Part model, mm, in its own coordinate system. A direction names the side the tool comes from. Give positions to 0.01 mm unless a question says otherwise; leave off trailing zeros. Order: outer loops, then holes, each group sorted by start corner. A loop starts at its lowest first (then second) coordinate and runs counter-clockwise, first axis right, second up. Notation, with made-up numbers: (75, 60.25) - (116, 60.25) arc R24 ccw to (116, 94.25) - close; hole circle Ø7 at (-2.5, 62). An arc over 180 degrees is marked (long way). One line per item, written item: value.
```python
from build123d import *

# Parameters (mm, degrees)
F1_DEPTH = 63.5
F2_DEPTH = 25.4
F3_DEPTH = 7.9375
F5_R     = 6.35


with BuildPart() as f1:
    # F0 (on Front) → F1 (new body, symmetric)
    with BuildSketch(Plane.XZ):
        Polygon((-41.275, 9.525), (-41.275, -9.525), (41.275, -9.525), (41.275, 9.525), (22.225, 9.525), align=None)
    extrude(amount=F1_DEPTH, both=True)

    # F0 (on Front) → F2 (join, symmetric)
    with BuildSketch(Plane.XZ):
        with BuildLine():
            Line((22.225, 9.525), (41.275, 9.525))
            Line((41.275, 9.525), (41.275, 30.6455698351))
            ThreePointArc((41.275, 30.6455698351), (44.8569757439, 39.2932242561), (53.5046301649, 42.8752))
            Line((53.5046301649, 42.8752), (60.325, 42.8752))
            Line((60.325, 42.8752), (60.325, 61.9252))
            Line((60.325, 61.9252), (53.5046301649, 61.9252))
            add(Edge.make_bspline(
                [(51.2267353125, 61.8421475047), (51.9857307237, 61.8741703131), (52.7450911942, 61.9018592787), (53.5046301649, 61.9252)],
                knots=[106.5779912672, 106.5779912672, 106.5779912672, 106.5779912672, 108.3003197328, 108.3003197328, 108.3003197328, 108.3003197328], degree=3))
            ThreePointArc((51.2267353125, 61.8421475047), (30.595385614, 51.943029246), (22.225, 30.6455698351))
            Line((22.225, 30.6455698351), (22.225, 9.525))
        make_face()
    extrude(amount=F2_DEPTH, both=True)

    # F0 (on Front) → F3 (join, symmetric)
    with BuildSketch(Plane.XZ):
        with BuildLine():
            add(Edge.make_bspline(
                [(-41.275, 9.525), (-41.3089372245, 41.2840319087), (4.2599645019, 59.8605704357), (51.2267353125, 61.8421475047)],
                knots=[0, 0, 0, 0, 106.5779912672, 106.5779912672, 106.5779912672, 106.5779912672], degree=3))
            Line((-41.275, 9.525), (22.225, 9.525))
            Line((22.225, 9.525), (22.225, 30.6455698351))
            ThreePointArc((22.225, 30.6455698351), (30.595385614, 51.943029246), (51.2267353125, 61.8421475047))
        make_face()
    extrude(amount=F3_DEPTH, both=True)

    # F0 (on Front) → F4 (revolve)
    with BuildSketch(Plane.XZ):
        Polygon((85.8790065383, 61.9252), (60.325, 61.9252), (60.325, 42.8752), (85.7558669821, 42.8752), align=None)
    revolve(axis=Axis((60.325, 0, 52.3875), (0, 0, 1)))

    # F5
    f5_edges = [f1.edges().sort_by_distance(p)[0] for p in [
        (-41.275, -63.5, 0),
        (41.275, -63.5, 0),
        (41.275, 63.5, 0),
        (-41.275, 63.5, 0),
    ]]
    fillet(f5_edges, radius=F5_R)


solid = f1.part
```
1) Wall check: line 1 along Z through (x, y) = (3.5, 17) (3 decimals); line 2 along Y through (x, z) = (43, 59.5); line 3 along Z through (x, y) = (59, -5.5). Give the ranges that are in metal, low to high. Write a range as [from, to].
Answer:
line 1: z = [-9.525, 9.525]
line 2: y = [-25.4, 25.4]
line 3: z = [42.88, 61.93]
2) Slice it at A-A on y = -50. Write the cut outline in (x, z) (3 decimals), then the cut area to 3 significant figures.
Answer:
outline: (-41.275, -9.525) - (41.275, -9.525) - (41.275, 9.525) - (-41.275, 9.525) - close
area: 1,570 mm2
3) Drop flat-ended pins along their axis: P1, Ø8.5, axis at y = -14, z = 23.5, coming from the -X side (3 decimals); P2, Ø8, axis at x = 11.5, z = 28.5, coming from the +Y side; P3, Ø10, axis at x = 28, y = -4.5, coming from the +Z side. Give the stop position or say it passes through.
Answer:
P1: stops at x = 22.225
P2: stops at y = 7.94
P3: stops at z = 60.22
4) Which spindle directions (+Z, -Z, +X, -X, +Y, -Y) get a long thin tool onto all of the face, cutting with end or side? Do faces 1 (the face through (22.225, -17, 20)), 2 (the face through (66, 0, 42.875)), 3 (the face through (39.365, 61.689, 0.133)), 4 (the face through (27.57, 16.55, 48.13)), 5 (the face through (0, 63.5, 0)). Say none if no direction does.
Answer:
face 1: +Z, -X, -Y
face 2: -Z, +X, +Y, -Y
face 3: +Z, -Z, +X, +Y
face 4: +Z, -X, +Y
face 5: +Z, -Z, +X, -X, +Y
